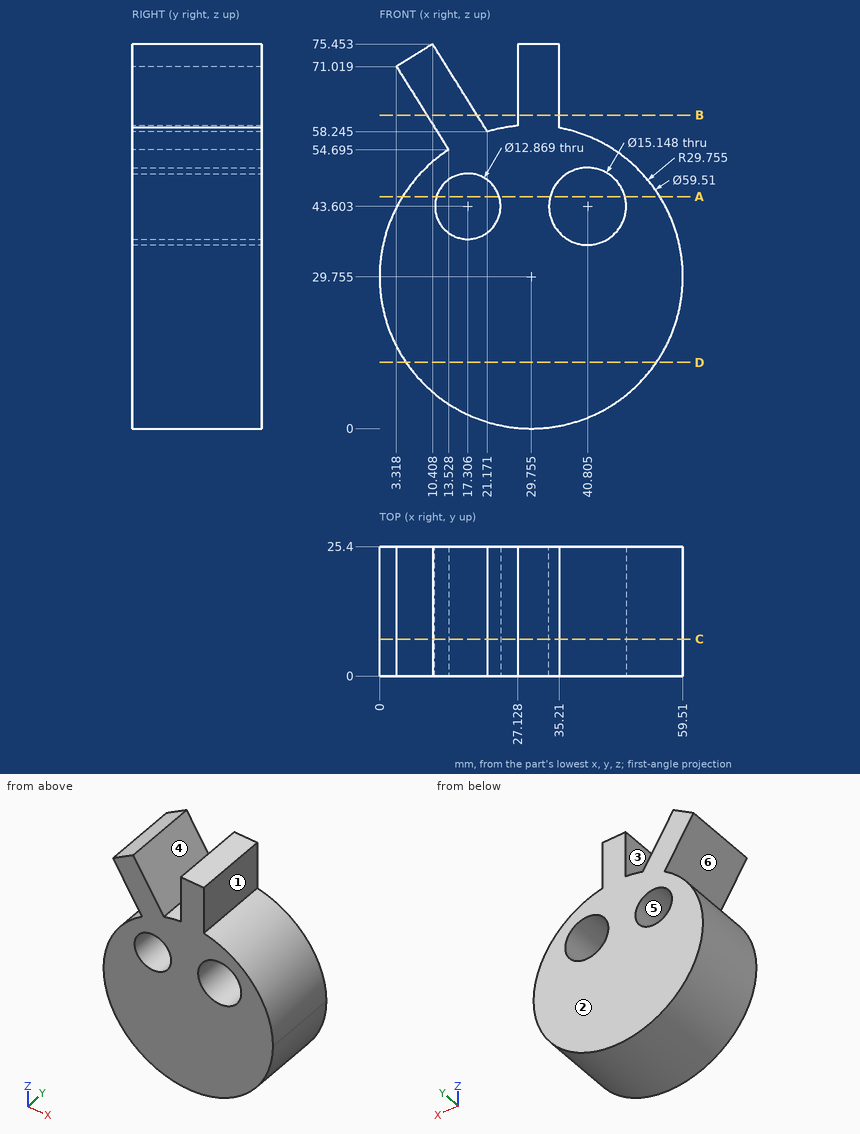
Could you check a few things on this drawing? It's one solid part, dimensions in mm from its lowest x, y, z. A direction names the side the tool comes from. Give positions to 0.01 mm unless a question says otherwise; leave off trailing zeros. Order: outer loops, then holes, each group sorted by start corner. A loop starts at its lowest first (then second) coordinate and runs counter-clockwise, first axis right, second up. Notation, with made-up numbers: (5, 45) - (20, 45) arc R16 cw to (20, 55) - close; hole circle Ø6 at (6.25, 86.5). An arc over 180 degrees is marked (long way). Answer as a JSON object with one key per item and string values. Group by question number.
Item 1: If we section it at D-D on z = 13: Please give me the cut outline in (x, y) (1 decimal), and give its area (3 significant figures).
Item 2: If we section it at A-A on z = 45.5: Please give me the cut outline in (x, y).
Item 3: For P1, Ø5, axis at y = 18, z = 65.5, coming from the -X side (1 decimal); P2, Ø4, axis at y = 6.5, z = 35, coming from the -X side; P3, Ø1.5, axis at y = 13.5, z = 65, coming from the +X side, each with a flat end and sliding along its axis, tell me the tip position at first contact or that it passes through.
Item 4: Please list where these lines run through material, in increasing order: probe 1 along Z at (x, y) = (10.5, 22.25) (1 decimal); probe 2 along Z at (x, y) = (18, 22) (1 decimal); probe 3 along X at (y, z) = (8.75, 60) (1 decimal).
Item 5: If we section it at B-B on z = 61.5: Please give me the cut outline in (x, y) (1 decimal).
Item 6: If we section it at C-C on y = 7.25: Please give me the cut outline in (x, z) (1 decimal).
Item 7: Which directions (+Z, -Z, +X, -X, +Y, -Y) give clear straight access to the entire face, cutting with the end or side of a thin tool? Please do the marked faces 4, 5 and 6.
Item 8: If we mould it in two halves opening along X, with no side actions, what happens to the marked faces 1, 2 and 3? For each: pulls with the +X half, pulls with the -X half, needs draft (parallel to the pull), parting line crosses it, or undercut.
Result set:
{
 "1": {"outline": "(5.2, 0) - (54.3, 0) - (54.3, 25.4) - (5.2, 25.4) - close", "area": "1,250 mm²"},
 "2": {"outline": "(4.51, 0) - (11.16, 0) - (11.16, 25.4) - (4.51, 25.4) - close; (23.45, 0) - (33.47, 0) - (33.47, 25.4) - (23.45, 25.4) - close; (48.14, 0) - (55, 0) - (55, 25.4) - (48.14, 25.4) - close"},
 "3": {"P1": "x = 5.2", "P2": "x = 0.18", "P3": "x = 35.21"},
 "4": {"probe 1": "7.1 to 52.4, 59.5 to 75.3", "probe 2": "2.4 to 37.2, 50 to 63.3", "probe 3": "10.2 to 20.1, 27.1 to 35.2"},
 "5": {"outline": "(9.3, 0) - (19.1, 0) - (19.1, 25.4) - (9.3, 25.4) - close; (27.1, 0) - (35.2, 0) - (35.2, 25.4) - (27.1, 25.4) - close"},
 "6": {"outline": "(3.3, 71) - (13.5, 54.7) arc R29.8 ccw (long way) to (59.5, 29.8) arc R29.8 ccw to (35.2, 59) - (35.2, 75.5) - (27.1, 75.5) - (27.1, 59.4) arc R29.8 ccw to (21.2, 58.2) - (10.4, 75.5) - close; hole circle Ø12.9 at (17.3, 43.6); hole circle Ø15.1 at (40.8, 43.6)"},
 "7": {"face 4": "+Z, +Y, -Y", "face 5": "+Y, -Y", "face 6": "-X, +Y, -Y"},
 "8": {"face 1": "pulls with the +X half", "face 2": "needs draft", "face 3": "undercut"}
}
